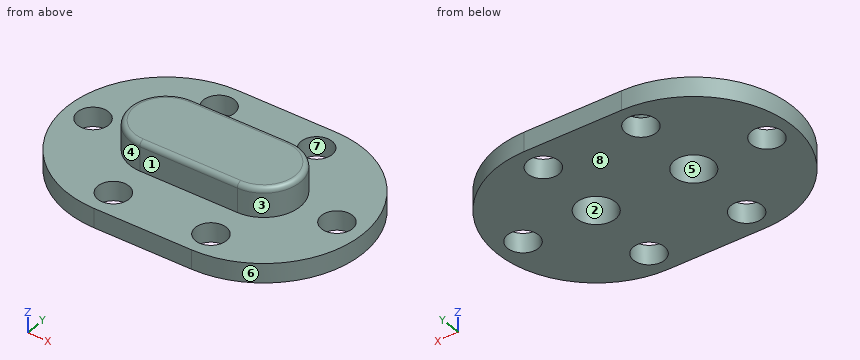
```python
from build123d import *

# Parameters (mm, degrees)
EXTRUDE_1_DEPTH           = 4
EXTRUDE_2_DEPTH           = 6
HOLE_WIZARD_8_0_8_1_D     = 8
HOLE_WIZARD_8_0_8_1_DEPTH = 7
HOLE_WIZARD_8_0_8_1_TIP   = 2.403442476
FILLET_2_R                = 1
SKETCH_10_R               = 3.203547284
CUT_EXTRUDE_1_DEPTH       = 38.235735524
PATTERN_CIRCULAR_1_COUNT  = 3
PATTERN_CIRCULAR_1_ANGLE  = 180
MIRROR_1_COPY_1_SKETCH_R  = 3.203547284
MIRROR_1_COPY_1_DEPTH     = 38.235735524
MIRROR_1_COPY_2_SKETCH_R  = 3.203547284
MIRROR_1_COPY_2_DEPTH     = 38.235735524


with BuildPart() as part:
    # 草图1 → 凸台-拉伸1 (new body)
    with BuildSketch(Plane.XY):
        with BuildLine():
            Line((-10, 20.5), (10, 20.5))
            ThreePointArc((10, 20.5), (30.5, 0), (10, -20.5))
            Line((10, -20.5), (-10, -20.5))
            ThreePointArc((-10, -20.5), (-30.5, 0), (-10, 20.5))
        make_face()
    extrude(amount=EXTRUDE_1_DEPTH)

    # 草图2 → 凸台-拉伸2 (add)
    with BuildSketch(Plane.XY.offset(4)):
        with BuildLine():
            Line((-10, 7.5), (10, 7.5))
            ThreePointArc((10, 7.5), (17.5, 0), (10, -7.5))
            Line((10, -7.5), (-10, -7.5))
            ThreePointArc((-10, -7.5), (-17.5, 0), (-10, 7.5))
        make_face()
    extrude(amount=EXTRUDE_2_DEPTH)

    # Ø8.0 (8) 直径孔1
    with Locations(Plane(origin=(0, 0, 0), x_dir=(-1, 0, 0), z_dir=(0, 0, -1))):
        with Locations((-10, 0), (10, 0)):
            Hole(HOLE_WIZARD_8_0_8_1_D / 2, depth=HOLE_WIZARD_8_0_8_1_DEPTH)
            with Locations((0, 0, -(HOLE_WIZARD_8_0_8_1_DEPTH + HOLE_WIZARD_8_0_8_1_TIP / 2))):  # 118° drill point
                Cone(0, HOLE_WIZARD_8_0_8_1_D / 2, HOLE_WIZARD_8_0_8_1_TIP, mode=Mode.SUBTRACT)

    # 圆角2
    fillet_2_edges = [part.edges().sort_by_distance(p)[0] for p in [
        (-17.5, 0, 10),
        (0, -7.5, 10),
        (17.5, 0, 10),
        (0, 7.5, 10),
    ]]
    fillet(fillet_2_edges, radius=FILLET_2_R)

    # 草图10 → 切除-拉伸1 (cut, symmetric)
    with BuildSketch(Plane.XY.offset(4)):
        with Locations((-10, 15)):
            Circle(SKETCH_10_R)
    cut_extrude_1 = extrude(amount=CUT_EXTRUDE_1_DEPTH, both=True, mode=Mode.SUBTRACT)

    # 阵列(圆周)1: 切除-拉伸1 ×3 about axis
    pattern_circular_1_axis = Axis((-10, 0, 0), (0, 0, 1))
    for i in range(1, PATTERN_CIRCULAR_1_COUNT):
        add(cut_extrude_1.rotate(pattern_circular_1_axis, i * PATTERN_CIRCULAR_1_ANGLE / (PATTERN_CIRCULAR_1_COUNT - 1)), mode=Mode.SUBTRACT)

    # 镜向1: 切除-拉伸1 across plane
    add(cut_extrude_1.mirror(Plane(origin=(0, 0, 0), x_dir=(0, 0, 1), z_dir=(1, 0, 0))), mode=Mode.SUBTRACT)

    # 镜向1 copy 1 sketch → 镜向1 copy 1 (cut, symmetric)
    with BuildSketch(Plane(origin=(10, 10, 4), x_dir=(0, 1, 0), z_dir=(0, 0, 1))):
        with Locations((-10, -15)):
            Circle(MIRROR_1_COPY_1_SKETCH_R)
    extrude(amount=MIRROR_1_COPY_1_DEPTH, both=True, mode=Mode.SUBTRACT)

    # 镜向1 copy 2 sketch → 镜向1 copy 2 (cut, symmetric)
    with BuildSketch(Plane(origin=(20, 0, 4), x_dir=(1, 0, 0), z_dir=(0, 0, 1))):
        with Locations((-10, -15)):
            Circle(MIRROR_1_COPY_2_SKETCH_R)
    extrude(amount=MIRROR_1_COPY_2_DEPTH, both=True, mode=Mode.SUBTRACT)


solid = part.part
```
Geometry: final body of the model. Coordinates: model frame, mm. Face numbers are marked on the shaded views. A direction names the side the tool comes from. Round coordinates to 2 decimals unless told otherwise and drop trailing zeros. Write each loop counter-clockwise with the first axis right and the second up, starting at its lowest first coordinate (ties: lowest second). Pieces come first, ordered by that corner, then holes. Notation, with made-up numbers: M 85.25,55 L 97.25,55 A29 cw 97.25,82 Z; hole C 23,34 d5. An arc over 180 degrees is marked long. Answer in a Markdown table with one row per item. Add a question column.
(1) Cut plane C-C, the plane x = -25. Return the cut outline in (y, z), then the cut area to 3 significant figures.
(2) Cut plane A-A, the plane z = 3.25. Give the number of separate pieces and of enclosed holes in the cut face, then the cut area to 3 significant figures.
(3) Contact query for flat-ended pins moving along their axis: pin 1 (5.5 mm diameter, centred on x = 1.5, z = 7, fed in from +Y); pin 2 (3 mm diameter, centred on x = -16, z = 7.5, fed in from +Y); pin 3 (6 mm diameter, centred on x = -25, y = 0, fed in from +Z); pin 4 (6 mm diameter, centred on x = -16.5, z = 8, fed in from +Y). Output: stop coordinate, or through.
(4) Cut plane B-B, the plane y = 15. Return the cut outline in (x, z).
(5) Ray query, L1, parallel to X at y = 0, z = 3; L2, parallel to Y at x = 10, z = 3; L3, parallel to Y at x = -10, z = 4.25. Return the intervals inside material, ascending.
(6) Reachability of the marked faces 1, 2, 3 and 4 from +Z, -Z, +X, -X, +Y, -Y: full face, straight path, thin tool, end or side. Return the list, or none.
(7) Draft query along X for the marked faces 5, 6, 7 and 8. Return one class per face: pulls with the +X half, pulls with the -X half, needs draft (parallel to the pull), parting line crosses it, or undercut.
(8) Cut plane D-D, the plane x = -1. Return the cut outline in (y, z).
Established:
| question | item | result |
|---|---|---|
| 1 | outline | M -13.97,0 L -3.2,0 L -3.2,4 L -13.97,4 Z; M 3.2,0 L 13.97,0 L 13.97,4 L 3.2,4 Z |
| 1 | area | 86.2 mm² |
| 2 | separate pieces | 1 |
| 2 | enclosed holes | 8 |
| 2 | area | 1,850 mm² |
| 3 | pin 1 | y = 7.5 |
| 3 | pin 2 | y = 6 |
| 3 | pin 3 | through |
| 3 | pin 4 | y = 6.63 |
| 4 | outline | M -23.97,0 L -13.2,0 L -13.2,4 L -23.97,4 Z; M -6.8,0 L 6.8,0 L 6.8,4 L -6.8,4 Z; M 13.2,0 L 23.97,0 L 23.97,4 L 13.2,4 Z |
| 5 | L1 | -30.5 to -28.2, -21.8 to -14, -6 to 6, 14 to 21.8, 28.2 to 30.5 |
| 5 | L2 | -20.5 to -18.2, -11.8 to -4, 4 to 11.8, 18.2 to 20.5 |
| 5 | L3 | -7.5 to -4, 4 to 7.5 |
| 6 | face 1 | +Z, +X, -X, -Y |
| 6 | face 2 | -Z |
| 6 | face 3 | +Z, +X |
| 6 | face 4 | +Z, -X |
| 7 | face 5 | undercut |
| 7 | face 6 | pulls with the +X half |
| 7 | face 7 | undercut |
| 7 | face 8 | needs draft |
| 8 | outline | M -20.5,0 L 20.5,0 L 20.5,4 L 7.5,4 L 7.5,9 A1 ccw 6.5,10 L -6.5,10 A1 ccw -7.5,9 L -7.5,4 L -20.5,4 Z |
